```python
from build123d import *

# Parameters (mm, degrees)
BOSS_EXTRUDE1_DEPTH = 2
SKETCH3_W           = 20
SKETCH3_H           = 87.5
BOSS_EXTRUDE4_DEPTH = 2
CIRPATTERN1_COUNT   = 2
CIRPATTERN1_ANGLE   = 90
CHAMFER1_DEPTH      = 2
SKETCH5_R           = 1.5
BOSS_EXTRUDE6_DEPTH = 2
CHAMFER3_SIZE       = 1


with BuildPart() as part:
    # Sketch1 → Boss-Extrude1 (new body)
    with BuildSketch(Plane(origin=(0, 0, 0), x_dir=(1, 0, 0), z_dir=(0, 1, 0))):
        Polygon((53.75, 5.29391293), (51.684417643, 15.678296686), (47.632632102, 25.460172293), (41.750351221, 34.263627757), (34.263627757, 41.750351221), (25.460172293, 47.632632102), (15.678296686, 51.684417643), (5.29391293, 53.75), (-5.29391293, 53.75), (-15.678296686, 51.684417643), (-25.460172293, 47.632632102), (-34.263627757, 41.750351221), (-41.750351221, 34.263627757), (-47.632632102, 25.460172293), (-51.684417643, 15.678296686), (-53.75, 5.29391293), (-53.75, -5.29391293), (-51.684417643, -15.678296686), (-47.632632102, -25.460172293), (-41.750351221, -34.263627757), (-34.263627757, -41.750351221), (-25.460172293, -47.632632102), (-15.678296686, -51.684417643), (-5.29391293, -53.75), (5.29391293, -53.75), (15.678296686, -51.684417643), (25.460172293, -47.632632102), (34.263627757, -41.750351221), (41.750351221, -34.263627757), (47.632632102, -25.460172293), (51.684417643, -15.678296686), (53.75, -5.29391293), align=None)
        Polygon((43.75, 4.308998897), (42.068712035, 12.76140428), (38.770747059, 20.723396052), (33.982844017, 27.888999337), (27.888999337, 33.982844017), (20.723396052, 38.770747059), (12.76140428, 42.068712035), (4.308998897, 43.75), (-4.308998897, 43.75), (-12.76140428, 42.068712035), (-20.723396052, 38.770747059), (-27.888999337, 33.982844017), (-33.982844017, 27.888999337), (-38.770747059, 20.723396052), (-42.068712035, 12.76140428), (-43.75, 4.308998897), (-43.75, -4.308998897), (-42.068712035, -12.76140428), (-38.770747059, -20.723396052), (-33.982844017, -27.888999337), (-27.888999337, -33.982844017), (-20.723396052, -38.770747059), (-12.76140428, -42.068712035), (-4.308998897, -43.75), (4.308998897, -43.75), (12.76140428, -42.068712035), (20.723396052, -38.770747059), (27.888999337, -33.982844017), (33.982844017, -27.888999337), (38.770747059, -20.723396052), (42.068712035, -12.76140428), (43.75, -4.308998897), align=None, mode=Mode.SUBTRACT)
    extrude(amount=BOSS_EXTRUDE1_DEPTH)

    # Sketch3 → Boss-Extrude4 (add)
    with BuildSketch(Plane(origin=(0, 2, 0), x_dir=(1, 0, 0), z_dir=(0, 1, 0))):
        Rectangle(SKETCH3_W, SKETCH3_H)
    boss_extrude4 = extrude(amount=-BOSS_EXTRUDE4_DEPTH)

    # CirPattern1: Boss-Extrude4 ×2 about axis
    cirpattern1_axis = Axis((0, 2, 0), (0, 1, 0))
    for i in range(1, CIRPATTERN1_COUNT):
        add(boss_extrude4.rotate(cirpattern1_axis, i * CIRPATTERN1_ANGLE / (CIRPATTERN1_COUNT - 1)))

    # Chamfer1: read off the stored shape, not the designer's step
    # Chamfer1 outline → Chamfer1 (add)
    with BuildSketch(Plane(origin=(0, 0, 0), x_dir=(1, 0, 0), z_dir=(0, 1, 0))):
        Polygon((10, -10), (10, -14), (14, -10), align=None)
        Polygon((13.692057296, -41.683222934), (10, -39.216269119), (10, -42.617989498), (12.76140428, -42.068712035), align=None)
        Polygon((42.617989498, -10), (39.216269119, -10), (41.683222934, -13.692057296), (42.068712035, -12.76140428), align=None)
        Polygon((-10, 10), (-10, 14), (-14, 10), align=None)
        Polygon((-13.692057296, 41.683222934), (-10, 39.216269119), (-10, 42.617989498), (-12.76140428, 42.068712035), align=None)
        Polygon((-42.617989498, 10), (-39.216269119, 10), (-41.683222934, 13.692057296), (-42.068712035, 12.76140428), align=None)
        Polygon((10, 10), (14, 10), (10, 14), align=None)
        Polygon((41.683222934, 13.692057296), (39.216269119, 10), (42.617989498, 10), (42.068712035, 12.76140428), align=None)
        Polygon((10, 42.617989498), (10, 39.216269119), (13.692057296, 41.683222934), (12.76140428, 42.068712035), align=None)
        Polygon((-10, -10), (-14, -10), (-10, -14), align=None)
        Polygon((-41.683222934, -13.692057296), (-39.216269119, -10), (-42.617989498, -10), (-42.068712035, -12.76140428), align=None)
        Polygon((-10, -42.617989498), (-10, -39.216269119), (-13.692057296, -41.683222934), (-12.76140428, -42.068712035), align=None)
    extrude(amount=CHAMFER1_DEPTH)

    # Sketch5 → Boss-Extrude6 (add)
    # profile 1 of 3: a face of its own
    with BuildSketch(Plane(origin=(0, 2, 0), x_dir=(1, 0, 0), z_dir=(0, 1, 0))):
        Polygon((-54.729274058, 3.5), (-58.770725942, 3.5), (-60.791451884, 0), (-58.770725942, -3.5), (-54.729274058, -3.5), (-53.75, -3.5), (-53.75, 3.5), align=None)
        with Locations(Location((-56.75, 0, 0), (0, 0, 270))):
            Circle(SKETCH5_R, mode=Mode.SUBTRACT)
    # profile 2 of 3: a face of its own
    with BuildSketch(Plane(origin=(0, 2, 0), x_dir=(1, 0, 0), z_dir=(0, 1, 0))):
        Polygon((54.729274058, 3.5), (53.75, 3.5), (53.75, -3.5), (54.729274058, -3.5), (58.770725942, -3.5), (60.791451884, 0), (58.770725942, 3.5), align=None)
        with Locations(Location((56.75, 0, 0), (0, 0, 270))):
            Circle(SKETCH5_R, mode=Mode.SUBTRACT)
    # profile 3 of 3: a face of its own
    with BuildSketch(Plane(origin=(0, 2, 0), x_dir=(1, 0, 0), z_dir=(0, 1, 0))):
        Polygon((3.5, -54.729274058), (3.5, -53.75), (-3.5, -53.75), (-3.5, -54.729274058), (-3.5, -58.770725942), (0, -60.791451884), (3.5, -58.770725942), align=None)
        with Locations(Location((0, -56.75, 0), (0, 0, 270))):
            Circle(SKETCH5_R, mode=Mode.SUBTRACT)
    extrude(amount=-BOSS_EXTRUDE6_DEPTH)

    # Chamfer3
    chamfer3_edges = [part.edges().sort_by_distance(p)[0] for p in [
        (-53.75, 1, 3.5),
        (-53.75, 1, -3.5),
        (53.75, 1, -3.5),
        (53.75, 1, 3.5),
        (3.5, 1, 53.75),
        (-3.5, 1, 53.75),
    ]]
    chamfer(chamfer3_edges, length=CHAMFER3_SIZE)


solid = part.part
```
Here's how the part is built. I have some questions about the finished solid (model axes, mm). A direction names the side the tool comes from. Round coordinates to 2 decimals unless told otherwise and drop trailing zeros. Order: outer loops, then holes, each group sorted by start corner. A loop starts at its lowest first (then second) coordinate and runs counter-clockwise, first axis right, second up. Notation, with made-up numbers: M 84,12.5 L 121,12.5 A21 cw 121,40.5 Z; hole C -30.5,66.5 d3. An arc over 180 degrees is marked long. Answer in a Markdown table with one row per item.
Item 1: I'm going to push flat-ended pins straight in: pin 1 (1 mm diameter, centred on x = -21, y = 1, fed in from -Z); pin 2 (1 mm diameter, centred on x = 56, y = 0.5, fed in from +Z); pin 3 (1 mm diameter, centred on y = 1.5, z = 24.5, fed in from +X). Where does each tip first touch, or does it pass through?
A:
| item | result |
|---|---|
| pin 1 | stops at z = -49.69 |
| pin 2 | stops at z = 3.5 |
| pin 3 | stops at x = 48.24 |
Item 2: Imagine slicing it at A-A, the plane z = 56.75. Write out the boundary of the cut face in (x, y), and give its area (3 significant figures).
A:
| item | result |
|---|---|
| outline | M -3.5,0 L -1.5,0 L -1.5,2 L -3.5,2 Z; M 1.5,0 L 3.5,0 L 3.5,2 L 1.5,2 Z |
| area | 8.00 mm2 |
Item 3: Imagine slicing it at D-D, the plane y = 0.6. State how many separate pieces and enclosed holes the cut face has, and give its area (3 significant figures).
A:
| item | result |
|---|---|
| separate pieces | 1 |
| enclosed holes | 7 |
| area | 6,340 mm2 |
Item 4: Thinking about a two-plate mould opening in X: for faces 1 (the face through (30.98, 0.99, -30.89)), 2 (the face through (44.733, 0.986, -29.8)), 3 (the face through (-1, 0, 3)), which applies, +X half, -X half, draft (parallel to the pull), parting line (faces both ways), or undercut?
A:
| item | result |
|---|---|
| face 1 | undercut |
| face 2 | +X half |
| face 3 | draft |
Item 5: For faces 4 (the face through (30.89, 0.99, 30.98)), 5 (the face through (-38.059, 0.986, 37.955)), which set-ups out of +Z, -Z, +X, -X, +Y, -Y let a thin tool reach every point of the face, with its end or its side?
A:
| item | result |
|---|---|
| face 4 | +Y, -Y |
| face 5 | +Z, -X, +Y, -Y |
Item 6: Imagine slicing it at C-C, the plane z = 36.5. Write out the boundary of the cut face in (x, y), and give its area (3 significant figures).
A:
| item | result |
|---|---|
| outline | M -39.51,0 L -24.12,0 L -24.12,2 L -39.51,2 Z; M -10,0 L 10,0 L 10,2 L -10,2 Z; M 24.12,0 L 39.51,0 L 39.51,2 L 24.12,2 Z |
| area | 102 mm2 |
Item 7: Imagine slicing it at B-B, the plane x = 56.75. Write out the boundary of the cut face in (y, z), and give its area (3 significant figures).
A:
| item | result |
|---|---|
| outline | M 0,-3.5 L 2,-3.5 L 2,-1.5 L 0,-1.5 Z; M 0,1.5 L 2,1.5 L 2,3.5 L 0,3.5 Z |
| area | 8.00 mm2 |
Item 8: If I drill on L1, parallel to X at y = 0.55, z = 0; L2, parallel to Z at x = 41, y = 0.35; L3, parallel to Z at x = 25, y = 1.55, over which ranges is the centre line in solid material (lowest first)? Write a range as from..to.
A:
| item | result |
|---|---|
| L1 | x = -60.79..-58.25, -55.25..55.25, 58.25..60.79 |
| L2 | z = -35.01..-15.34, -12.67..12.67, 15.34..35.01 |
| L3 | z = -47.82..-35.91, -10..10, 35.91..47.82 |
